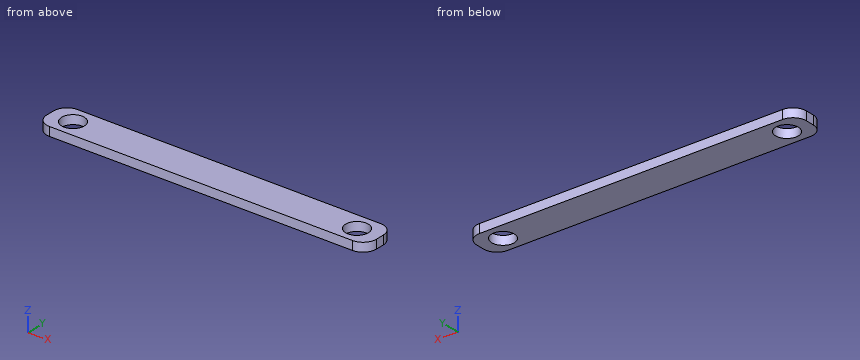
from build123d import *

# Parameters (mm, degrees)
SKETCH1_W           = 185.8
SKETCH1_H           = 20
SKETCH1_R           = 6.45
BOSS_EXTRUDE1_DEPTH = 5
FILLET1_R           = 7.5


with BuildPart() as part:
    # Sketch1 → Boss-Extrude1 (new body)
    with BuildSketch(Plane.XY):
        Rectangle(SKETCH1_W, SKETCH1_H)
        with Locations((-80, 0)):
            Circle(SKETCH1_R, mode=Mode.SUBTRACT)
        with Locations((80, 0)):
            Circle(SKETCH1_R, mode=Mode.SUBTRACT)
    extrude(amount=BOSS_EXTRUDE1_DEPTH)

    # Fillet1
    fillet1_edges = [part.edges().sort_by_distance(p)[0] for p in [
        (-92.9, 10, 2.5),
        (92.9, 10, 2.5),
        (92.9, -10, 2.5),
        (-92.9, -10, 2.5),
    ]]
    fillet(fillet1_edges, radius=FILLET1_R)


solid = part.part
Model file for the job. Use its own axes, mm. Give positions to 0.01 mm unless a question says otherwise; leave off trailing zeros. Order: outer loops, then holes, each group sorted by start corner. A loop starts at its lowest first (then second) coordinate and runs counter-clockwise, first axis right, second up. Notation, with made-up numbers: (34.25, 35) - (61.25, 35) arc R35 ccw to (61.25, 70) - close; hole circle Ø3 at (33.25, -23). An arc over 180 degrees is marked (long way). Return JSON: item names as keys, results as strings.
1) Cut at B-B, the plane x = -80. Give the cut face in (y, z), plus the area to 3 significant figures.
Geometry says:
{"outline": "(-10, 0) - (-6.45, 0) - (-6.45, 5) - (-10, 5) - close; (6.45, 0) - (10, 0) - (10, 5) - (6.45, 5) - close", "area": "35.5 mm²"}
2) Flat gauge pin, fed straight in: P1, Ø10, axis at x = -45.5, y = -7, coming from the -Z side. Where does the tip first touch, or does it go through?
Geometry says:
{"P1": "z = 0"}
3) Cut at C-C, the plane z = 3. Give the cut face in (x, y), plus the area to 3 significant figures.
Geometry says:
{"outline": "(-92.9, -2.5) arc R7.5 ccw to (-85.4, -10) - (85.4, -10) arc R7.5 ccw to (92.9, -2.5) - (92.9, 2.5) arc R7.5 ccw to (85.4, 10) - (-85.4, 10) arc R7.5 ccw to (-92.9, 2.5) - close; hole circle Ø12.9 at (-80, 0); hole circle Ø12.9 at (80, 0)", "area": "3,410 mm²"}
4) Cut at A-A, the plane y = 0. Give the cut face in (x, z), plus the area to 3 significant figures.
Geometry says:
{"outline": "(-92.9, 0) - (-86.45, 0) - (-86.45, 5) - (-92.9, 5) - close; (-73.55, 0) - (73.55, 0) - (73.55, 5) - (-73.55, 5) - close; (86.45, 0) - (92.9, 0) - (92.9, 5) - (86.45, 5) - close", "area": "800 mm²"}
5) Probe line 1 (Y direction, x = -80, z = 3.95); line 2 (X direction, y = 5.5, z = 3.05); line 3 (X direction, y = 4.25, z = 0.85). List the from-to ranges inside material, lowest first. Write a range as from..to.
Geometry says:
{"line 1": "-10..-6.45, 6.45..10", "line 2": "-92.27..-83.37, -76.63..76.63, 83.37..92.27", "line 3": "-92.69..-84.85, -75.15..75.15, 84.85..92.69"}
